from build123d import *

# Parameters (mm, degrees)
F0_W      = 147
F0_H      = 102
F1_DEPTH  = 26
F2_R      = 2
F3_R      = 25.1169689263
F4_DEPTH  = 3
F6_DEPTH  = 2
F7_R      = 25.1169689263
F7_W      = 7.9772167655
F7_H      = 4.1224605193
F7_W_2    = 4.1224605193
F7_H_2    = 7.9772167655
F8_DEPTH  = 2
F9_SIZE2  = 1.99999
F9_SIZE   = 6.99999
F10_R     = 5
F12_DEPTH = 2
F13_R     = 1


# Not quite as in the source:
# - a fillet or chamfer is up to 0.001 mm smaller than in the source, because OpenCascade refuses the exact size


with BuildPart() as f1:
    # F0 (on Top) → F1 (new body)
    with BuildSketch(Plane.XY):
        with Locations((73.5, 51)):
            Rectangle(F0_W, F0_H)
    extrude(amount=F1_DEPTH)

    # F2
    f2_edges = [f1.edges().sort_by_distance(p)[0] for p in [
        (0, 0, 13),
        (147, 0, 13),
        (147, 102, 13),
        (0, 102, 13),
    ]]
    fillet(f2_edges, radius=F2_R)

    # F3 (on face) → F4 (cut)
    with BuildSketch(Plane(origin=(0, 0, 0), x_dir=(1, 0, 0), z_dir=(0, 0, -1))):
        with BuildLine():
            Line((144, -3), (6.5606157295, -3))
            Line((6.5606157295, -3), (6.5606157295, 0))
            Line((6.5606157295, 0), (2, 0))
            ThreePointArc((2, 0), (0.5857864376, -0.5857864376), (0, -2))
            Line((0, -2), (0, -100))
            ThreePointArc((0, -100), (0.5857864376, -101.4142135624), (2, -102))
            Line((2, -102), (14.2296897247, -102))
            Line((14.2296897247, -102), (14.2296897247, -99))
            Line((14.2296897247, -99), (145, -99))
            Line((145, -99), (137.9531513453, -85.8632188108))
            Line((137.9531513453, -85.8632188108), (137.9531513453, -16.6260308719))
            Line((137.9531513453, -16.6260308719), (144, -3))
        make_face()
        with Locations((98.0989858508, -50.0876903534)):
            Circle(F3_R, mode=Mode.SUBTRACT)
        Polygon((147, -97.1357934826), (147, -3), (140.9531513453, -16.6260308719), (140.9531513453, -85.8632188108), align=None)
    extrude(amount=-F4_DEPTH, mode=Mode.SUBTRACT)

    # F5 (on face) → F6 (join)
    with BuildSketch(Plane(origin=(0, 0, 3), x_dir=(1, 0, 0), z_dir=(0, 0, -1))):
        with BuildLine():
            Line((14.2296897247, -99), (55.0723448396, -99))
            Line((55.0723448396, -99), (55.0723448396, -42.5031647924))
            Line((55.0723448396, -42.5031647924), (23.9577665925, -28.1695667654))
            Line((23.9577665925, -28.1695667654), (0, -28.1695667654))
            Line((0, -28.1695667654), (0, -100))
            ThreePointArc((0, -100), (0.5857864376, -101.4142135624), (2, -102))
            Line((2, -102), (14.2296897247, -102))
            Line((14.2296897247, -102), (14.2296897247, -99))
        make_face()
    extrude(amount=F6_DEPTH)

    # F7 (on face) → F8 (join)
    with BuildSketch(Plane(origin=(0, 0, 3), x_dir=(1, 0, 0), z_dir=(0, 0, -1))):
        Polygon((68.5814172029, -11.8443537503), (68.5814172029, -22.7281169246), (68.5814172029, -36.7360695054), (68.5814172029, -79.8824131489), (92.3246070743, -79.8824131489), (108.6435541511, -79.8824131489), (128.9916932583, -79.8824131489), (128.9916932583, -11.8443537503), align=None)
        with Locations((98.0989858508, -50.0876903534)):
            Circle(F7_R, mode=Mode.SUBTRACT)
        Polygon((68.5814172029, -36.7360695054), (68.5814172029, -22.7281169246), (61.3132603467, -22.7281169246), (61.3132603467, -26.8505774438), (61.3132603467, -32.6136089861), (61.3132603467, -36.7360695054), align=None)
        Polygon((108.6435541511, -79.8824131489), (92.3246070743, -79.8824131489), (92.3246070743, -85.6698147568), (96.4470675935, -85.6698147568), (104.5210936318, -85.6698147568), (108.6435541511, -85.6698147568), align=None)
        with Locations((57.3246519639, -24.7893471842)):
            Rectangle(F7_W, F7_H)
        with Locations((57.3246519639, -34.6748392458)):
            Rectangle(F7_W, F7_H)
        with Locations((94.3858373339, -89.6584231396)):
            Rectangle(F7_W_2, F7_H_2)
        with Locations((106.5823238914, -89.6584231396)):
            Rectangle(F7_W_2, F7_H_2)
    extrude(amount=F8_DEPTH)

    # F9 (size 7 and 2 in the source; OpenCascade refuses exactly that, so slightly less here)
    f9_edges = [f1.edges().sort_by_distance(p)[0] for p in [
        (53.336044, 24.789347, 1),
        (53.336044, 34.674839, 1),
        (94.385837, 93.647032, 1),
        (106.582324, 93.647032, 1),
    ]]
    f9_side = f1.faces().sort_by_distance((69.695664, 17.286235, 1))[0]
    chamfer(f9_edges, length=F9_SIZE, length2=F9_SIZE2, reference=f9_side)

    # F10
    f10_edges = [f1.edges().sort_by_distance(p)[0] for p in [
        (68.581417, 11.844354, 2),
        (128.991693, 11.844354, 2),
        (128.991693, 79.882413, 2),
        (68.581417, 79.882413, 2),
    ]]
    fillet(f10_edges, radius=F10_R)

    # F11 (on face) → F12 (cut)
    with BuildSketch(Plane.XY.offset(26)):
        with BuildLine():
            ThreePointArc((2, 102), (0.5857864376, 101.4142135624), (0, 100))
            Line((0, 100), (0, 2))
            ThreePointArc((0, 2), (0.5857864376, 0.5857864376), (2, 0))
            Line((2, 0), (145, 0))
            ThreePointArc((145, 0), (146.4142135624, 0.5857864376), (147, 2))
            Line((147, 2), (147, 100))
            ThreePointArc((147, 100), (146.4142135624, 101.4142135624), (145, 102))
            Line((145, 102), (2, 102))
        make_face()
        with BuildLine():
            Line((4.2258142494, 22.0722364937), (4.2258142494, 51))
            Line((4.2258142494, 51), (4.2258142494, 79.9277635063))
            ThreePointArc((4.2258142494, 79.9277635063), (4.9610816932, 83.691369578), (7.058760382, 86.9015242465))
            Line((7.058760382, 86.9015242465), (14.6935671534, 94.7479464908))
            ThreePointArc((14.6935671534, 94.7479464908), (17.9707371795, 96.986612342), (21.8606210208, 97.7741857506))
            Line((21.8606210208, 97.7741857506), (55.7528358207, 97.7741857506))
            ThreePointArc((55.7528358207, 97.7741857506), (57.3980089851, 97.6379277008), (58.9983485321, 97.2328668025))
            Line((58.9983485321, 97.2328668025), (80.9614386994, 89.6967750441))
            ThreePointArc((80.9614386994, 89.6967750441), (82.5617782464, 89.2917141458), (84.2069514108, 89.1554560959))
            Line((84.2069514108, 89.1554560959), (91.6838514243, 89.1554560959))
            ThreePointArc((91.6838514243, 89.1554560959), (94.5898246688, 90.0866332315), (96.4134075766, 92.533328295))
            Line((96.4134075766, 92.533328295), (96.5889555539, 93.0451646719))
            ThreePointArc((96.5889555539, 93.0451646719), (99.1419716248, 96.4705377609), (103.2103341671, 97.7741857506))
            Line((103.2103341671, 97.7741857506), (125.9630903806, 97.7741857506))
            ThreePointArc((125.9630903806, 97.7741857506), (129.5503496104, 97.1086150968), (132.660093946, 95.2004999942))
            Line((132.660093946, 95.2004999942), (139.4711893161, 89.0582969469))
            ThreePointArc((139.4711893161, 89.0582969469), (141.9111993671, 85.6958456652), (142.7741857506, 81.6319827033))
            Line((142.7741857506, 81.6319827033), (142.7741857506, 51))
            Line((142.7741857506, 51), (142.7741857506, 20.3680172967))
            ThreePointArc((142.7741857506, 20.3680172967), (141.9111993671, 16.3041543348), (139.4711893161, 12.9417030531))
            Line((139.4711893161, 12.9417030531), (132.660093946, 6.7995000058))
            ThreePointArc((132.660093946, 6.7995000058), (129.5503496104, 4.8913849032), (125.9630903806, 4.2258142494))
            Line((125.9630903806, 4.2258142494), (103.2103341671, 4.2258142494))
            ThreePointArc((103.2103341671, 4.2258142494), (99.1419716248, 5.5294622391), (96.5889555539, 8.9548353281))
            Line((96.5889555539, 8.9548353281), (96.4134075766, 9.466671705))
            ThreePointArc((96.4134075766, 9.466671705), (94.5898246688, 11.9133667685), (91.6838514243, 12.8445439041))
            Line((91.6838514243, 12.8445439041), (84.2069514108, 12.8445439041))
            ThreePointArc((84.2069514108, 12.8445439041), (82.5617782464, 12.7082858542), (80.9614386994, 12.3032249559))
            Line((80.9614386994, 12.3032249559), (58.9983485321, 4.7671331975))
            ThreePointArc((58.9983485321, 4.7671331975), (57.3980089851, 4.3620722992), (55.7528358207, 4.2258142494))
            Line((55.7528358207, 4.2258142494), (21.8606210208, 4.2258142494))
            ThreePointArc((21.8606210208, 4.2258142494), (17.9707371795, 5.013387658), (14.6935671534, 7.2520535092))
            Line((14.6935671534, 7.2520535092), (7.058760382, 15.0984757535))
            ThreePointArc((7.058760382, 15.0984757535), (4.9610816932, 18.308630422), (4.2258142494, 22.0722364937))
        make_face(mode=Mode.SUBTRACT)
        with BuildLine():
            ThreePointArc((99.0220627739, 38.1232459871), (98.3651864651, 37.8055751771), (98.0989858508, 37.1262089566))
            Line((98.0989858508, 37.1262089566), (98.0989858508, 25.9914626364))
            ThreePointArc((98.0989858508, 25.9914626364), (98.4066942145, 25.269844808), (99.1404504313, 24.9923226619))
            ThreePointArc((99.1404504313, 24.9923226619), (115.8593649014, 32.3273113028), (123.1943535423, 49.0462257729))
            ThreePointArc((123.1943535423, 49.0462257729), (122.9168313962, 49.7799819897), (122.1952135678, 50.0876903534))
            Line((122.1952135678, 50.0876903534), (111.0604672476, 50.0876903534))
            ThreePointArc((111.0604672476, 50.0876903534), (110.3811010271, 49.8214897391), (110.0634302171, 49.1646134303))
            ThreePointArc((110.0634302171, 49.1646134303), (106.584267225, 41.6024089792), (99.0220627739, 38.1232459871))
        make_face()
    extrude(amount=-F12_DEPTH, mode=Mode.SUBTRACT)

    # F13
    f13_edges = [f1.edges().sort_by_distance(p)[0] for p in [
        (141.911199, 85.695846, 26),
        (142.774186, 51, 26),
        (141.911199, 16.304154, 26),
        (136.065642, 9.870602, 26),
        (129.55035, 4.891385, 26),
        (114.586712, 4.225814, 26),
        (99.141972, 5.529462, 26),
        (96.501182, 9.210754, 26),
        (94.589825, 11.913367, 26),
        (87.945401, 12.844544, 26),
        (82.561778, 12.708286, 26),
        (69.979894, 8.535179, 26),
        (57.398009, 4.362072, 26),
        (38.806728, 4.225814, 26),
        (17.970737, 5.013388, 26),
        (10.876164, 11.175265, 26),
        (4.961082, 18.30863, 26),
        (4.225814, 51, 26),
        (4.961082, 83.69137, 26),
        (10.876164, 90.824735, 26),
        (17.970737, 96.986612, 26),
        (38.806728, 97.774186, 26),
        (57.398009, 97.637928, 26),
        (69.979894, 93.464821, 26),
        (82.561778, 89.291714, 26),
        (87.945401, 89.155456, 26),
        (94.589825, 90.086633, 26),
        (96.501182, 92.789246, 26),
        (99.141972, 96.470538, 26),
        (114.586712, 97.774186, 26),
        (129.55035, 97.108615, 26),
        (136.065642, 92.129398, 26),
        (106.584267, 41.602409, 26),
        (98.365186, 37.805575, 26),
        (98.098986, 31.558836, 26),
        (98.406694, 25.269845, 26),
        (115.859365, 32.327311, 26),
        (122.916831, 49.779982, 26),
        (116.62784, 50.08769, 26),
        (110.381101, 49.82149, 26),
    ]]
    fillet(f13_edges, radius=F13_R)


solid = f1.part
Could you check a few things on this model? Use its own coordinates, in mm. A direction names the side the tool comes from. Give positions to 0.01 mm unless a question says otherwise; leave off trailing zeros. Order: outer loops, then holes, each group sorted by start corner. A loop starts at its lowest first (then second) coordinate and runs counter-clockwise, first axis right, second up. Notation, with made-up numbers: (-22.75, -17) - (1.25, -17) arc R18 ccw to (1.25, 1) - close; hole circle Ø7 at (-13, 67.5). An arc over 180 degrees is marked (long way). Return JSON: item names as keys, results as strings. Group by question number.
Q1. Will these pins go through, and if not, where does the flat tip stop? pin 1 Ø1.5 at (y, z) = (54.5, 1) entering from +X; pin 2 Ø4 at (x, y) = (65.5, 80.5) entering from -Z; pin 3 Ø1 at (y, z) = (21, 1.5) entering from -X.
Q2. Please list where these lines run through material, in increasing order: line 1 along Z through (x, y) = (101, 84); line 2 along Z through (x, y) = (6.5, 18); line 3 along X through (y, z) = (82.5, 24.25). Write a range as [from, to].
Q3. Suppose I cut it at A-A, the plane y = 70. Please give me the cut outline in (x, z), and give its area (3 significant figures).
Q4. Thinking about a two-plate mould opening in X: for faces 6 (the face through (144, 49, 3)), 7 (the face through (10.93, 11.12, 24.51)), 8 (the face through (70.04, 93.14, 25.7)), which applies, pulls with the +X half, pulls with the -X half, needs draft (parallel to the pull), parting line crosses it, or undercut?
Q5. Which directions (+Z, -Z, +X, -X, +Y, -Y) give clear straight access to the entire face, cutting with the end or side of a thin tool? Please do faces 1 (the face through (6.561, 2, 1)), 2 (the face through (127.49, 13.27, 1.99)), 3 (the face through (143.934, 91.421, 1.479)), 4 (the face through (70.007, 13.348, 1.986)), 5 (the face through (115.67, 32.14, 24.51)).
Q6. Suppose I cut it at B-B, the plane x = 32.5. Please give me the cut outline in (y, z).
Resolved:
{
 "1": {"pin 1": "stops at x = 140.95", "pin 2": "stops at z = 3", "pin 3": "stops at x = 68.58"},
 "2": {"line 1": "z = [1, 26]", "line 2": "z = [3, 26]", "line 3": "x = [4.56, 142.74]"},
 "3": {"outline": "(0, 1) - (55.07, 1) - (55.07, 3) - (68.58, 3) - (68.58, 1) - (82.79, 1) - (82.79, 0) - (113.41, 0) - (113.41, 1) - (128.99, 1) - (128.99, 3) - (137.95, 3) - (137.95, 0) - (140.95, 0) - (140.95, 3) - (147, 3) - (147, 24) - (142.77, 24) - (142.77, 25) arc R1 ccw to (141.77, 26) - (5.23, 26) arc R1 ccw to (4.23, 25) - (4.23, 24) - (0, 24) - close", "area": "3,630 mm2"},
 "4": {"face 6": "needs draft", "face 7": "pulls with the -X half", "face 8": "undercut"},
 "5": {"face 1": "-Z, -X, -Y", "face 2": "-Z", "face 3": "-Z, +X", "face 4": "-Z, -X", "face 5": "+Z"},
 "6": {"outline": "(0, 0) - (3, 0) - (3, 3) - (32.1, 3) - (32.1, 1) - (99, 1) - (99, 0) - (102, 0) - (102, 24) - (97.77, 24) - (97.77, 25) arc R1 ccw to (96.77, 26) - (5.23, 26) arc R1 ccw to (4.23, 25) - (4.23, 24) - (0, 24) - close"}
}
